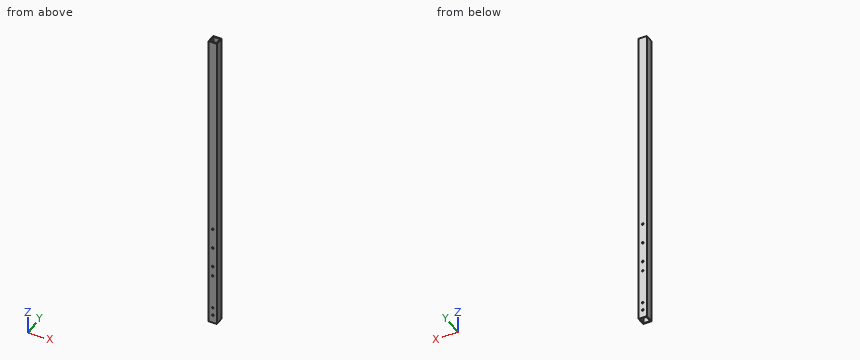
```python
from build123d import *

# Parameters (mm, degrees)
SKETCH_1_W          = 20
SKETCH_1_H          = 20
SKETCH_1_W_2        = 16
SKETCH_1_H_2        = 16
EXTRUDE_1_DEPTH     = 375
SKETCH_2_R          = 2
CUT_EXTRUDE_1_DEPTH = 376.666075125
SKETCH_3_R          = 2.25
CUT_EXTRUDE_2_DEPTH = 376.666075125


with BuildPart() as part:
    # 草图1 → 凸台-拉伸1 (new, symmetric)
    with BuildSketch(Plane.XY):
        Rectangle(SKETCH_1_W, SKETCH_1_H)
        Rectangle(SKETCH_1_W_2, SKETCH_1_H_2, mode=Mode.SUBTRACT)
    extrude(amount=EXTRUDE_1_DEPTH, both=True)

    # 草图2 → 切除-拉伸1 (cut, through all)
    with BuildSketch(Plane(origin=(0, 10, 0), x_dir=(1, 0, 0), z_dir=(0, 1, 0))):
        with Locations((0, 385)):
            Circle(SKETCH_2_R)
        with Locations(Location((0, 355, 0), (0, 0, 180))):
            Circle(SKETCH_2_R)
        with Locations(Location((0, 250, 0), (0, 0, 180))):
            Circle(SKETCH_2_R)
        with Locations(Location((0, 335, 0), (0, 0, 180))):
            Circle(SKETCH_2_R)
    extrude(amount=-CUT_EXTRUDE_1_DEPTH, mode=Mode.SUBTRACT)

    # 草图3 → 切除-拉伸2 (cut, through all)
    with BuildSketch(Plane(origin=(0, 10, 0), x_dir=(1, 0, 0), z_dir=(0, 1, 0))):
        with Locations(Location((0, 125, 0), (0, 0, 180))):
            Circle(SKETCH_3_R)
        with Locations(Location((0, 175, 0), (0, 0, 180))):
            Circle(SKETCH_3_R)
        with Locations(Location((0, 225, 0), (0, 0, 180))):
            Circle(SKETCH_3_R)
    extrude(amount=-CUT_EXTRUDE_2_DEPTH, mode=Mode.SUBTRACT)


solid = part.part
```
Can you work these out from the model? Positions are in its coordinate system, mm. Coordinates: 2 decimals unless noted, no trailing zeros. Order: outer loops, then holes, each group sorted by start corner. A loop starts at its lowest first (then second) coordinate and runs counter-clockwise, first axis right, second up.
1. If we section it at B-B (z = -299): Please give me the cut outline in (x, y), then the cut area to 3 significant figures.
2. If we section it at A-A (y = -1.5): Please give me the cut outline in (x, z).
3. I need wall thicknesses on line 1 (Y direction, x = -7, z = -162); line 2 (X direction, y = 9, z = -225). Which ranges of each line are inside material? Lowest first, please.
Entries:
1. outline: (-10, -10) - (10, -10) - (10, 10) - (-10, 10) - close; hole (-8, -8) - (8, -8) - (8, 8) - (-8, 8) - close
1. area: 144 mm2
2. outline: (-10, -375) - (-8, -375) - (-8, 375) - (-10, 375) - close; (8, -375) - (10, -375) - (10, 375) - (8, 375) - close
3. line 1: y = -10 to -8, 8 to 10
3. line 2: x = -10 to -2.25, 2.25 to 10
